from build123d import *

# Parameters (mm, degrees)
SKETCH1_W               = 350
SKETCH1_H               = 175
BOSS_EXTRUDE1_DEPTH     = 6
SKETCH3_W               = 6
SKETCH3_H               = 25
CUT_EXTRUDE1_DEPTH      = 392.357892472
LPATTERN1_COUNT         = 4
LPATTERN1_PITCH         = 50
SKETCH4_W               = 6
SKETCH4_H               = 10
CUT_EXTRUDE2_DEPTH      = 392.357892472
LPATTERN2_COUNT         = 2
LPATTERN2_PITCH         = 165
SKETCH5_W               = 6
SKETCH5_H               = 10
CUT_EXTRUDE3_DEPTH      = 392.357892472
LPATTERN3_COUNT         = 2
LPATTERN3_PITCH         = 165
SKETCH6_W               = 6
SKETCH6_H               = 50
CUT_EXTRUDE4_DEPTH      = 10
SKETCH7_W               = 20
SKETCH7_H               = 10
CUT_EXTRUDE5_DEPTH      = 10
LPATTERN4_COUNT         = 2
LPATTERN4_PITCH         = 165
SKETCH8_R               = 2.5
CUT_EXTRUDE6_DEPTH      = 10
SKETCH9_W               = 10
SKETCH9_H               = 20
CUT_EXTRUDE7_DEPTH      = 10
MIRROR1_COPY_1_SKETCH_W = 6
MIRROR1_COPY_1_SKETCH_H = 25
MIRROR1_COPY_1_DEPTH    = 392.357892472
MIRROR1_COPY_2_SKETCH_W = 6
MIRROR1_COPY_2_SKETCH_H = 25
MIRROR1_COPY_2_DEPTH    = 392.357892472
MIRROR1_COPY_3_SKETCH_W = 6
MIRROR1_COPY_3_SKETCH_H = 25
MIRROR1_COPY_3_DEPTH    = 392.357892472
MIRROR1_COPY_4_SKETCH_W = 6
MIRROR1_COPY_4_SKETCH_H = 10
MIRROR1_COPY_4_DEPTH    = 392.357892472
MIRROR1_COPY_5_SKETCH_W = 6
MIRROR1_COPY_5_SKETCH_H = 10
MIRROR1_COPY_5_DEPTH    = 392.357892472


with BuildPart() as part:
    # Sketch1 → Boss-Extrude1 (new body)
    with BuildSketch(Plane(origin=(0, 0, 0), x_dir=(0, 0, -1), z_dir=(1, 0, 0))):
        with Locations((-175, 87.5)):
            Rectangle(SKETCH1_W, SKETCH1_H)
    extrude(amount=BOSS_EXTRUDE1_DEPTH)

    # Sketch3 → Cut-Extrude1 (cut, through all)
    with BuildSketch(Plane(origin=(6, 0, 0), x_dir=(0, 0, -1), z_dir=(1, 0, 0))):
        with Locations((-297, 162.5)):
            Rectangle(SKETCH3_W, SKETCH3_H)
    cut_extrude1 = extrude(amount=-CUT_EXTRUDE1_DEPTH, mode=Mode.SUBTRACT)

    # LPattern1: Cut-Extrude1 ×4
    with Locations(*[(0, -i * LPATTERN1_PITCH, 0) for i in range(1, LPATTERN1_COUNT)]):
        add(cut_extrude1, mode=Mode.SUBTRACT)

    # Sketch4 → Cut-Extrude2 (cut, through all)
    with BuildSketch(Plane(origin=(6, 0, 0), x_dir=(0, 0, -1), z_dir=(1, 0, 0))):
        with Locations((-279, 170)):
            Rectangle(SKETCH4_W, SKETCH4_H)
    cut_extrude2 = extrude(amount=-CUT_EXTRUDE2_DEPTH, mode=Mode.SUBTRACT)

    # LPattern2: Cut-Extrude2 ×2
    with Locations(*[(0, -i * LPATTERN2_PITCH, 0) for i in range(1, LPATTERN2_COUNT)]):
        add(cut_extrude2, mode=Mode.SUBTRACT)

    # Sketch5 → Cut-Extrude3 (cut, through all)
    with BuildSketch(Plane(origin=(6, 0, 0), x_dir=(0, 0, -1), z_dir=(1, 0, 0))):
        with Locations((-249, 170)):
            Rectangle(SKETCH5_W, SKETCH5_H)
    cut_extrude3 = extrude(amount=-CUT_EXTRUDE3_DEPTH, mode=Mode.SUBTRACT)

    # LPattern3: Cut-Extrude3 ×2
    with Locations(*[(0, -i * LPATTERN3_PITCH, 0) for i in range(1, LPATTERN3_COUNT)]):
        add(cut_extrude3, mode=Mode.SUBTRACT)

    # Sketch6 → Cut-Extrude4 (cut)
    with BuildSketch(Plane(origin=(6, 0, 0), x_dir=(0, 0, -1), z_dir=(1, 0, 0))):
        with Locations((-175, 150)):
            Rectangle(SKETCH6_W, SKETCH6_H)
    extrude(amount=-CUT_EXTRUDE4_DEPTH, mode=Mode.SUBTRACT)

    # Sketch7 → Cut-Extrude5 (cut)
    with BuildSketch(Plane(origin=(6, 0, 0), x_dir=(0, 0, -1), z_dir=(1, 0, 0))):
        with Locations((-212, 170)):
            Rectangle(SKETCH7_W, SKETCH7_H)
    cut_extrude5 = extrude(amount=-CUT_EXTRUDE5_DEPTH, mode=Mode.SUBTRACT)

    # LPattern4: Cut-Extrude5 ×2
    with Locations(*[(0, -i * LPATTERN4_PITCH, 0) for i in range(1, LPATTERN4_COUNT)]):
        add(cut_extrude5, mode=Mode.SUBTRACT)

    # Sketch8 → Cut-Extrude6 (cut)
    with BuildSketch(Plane(origin=(6, 0, 0), x_dir=(0, 0, -1), z_dir=(1, 0, 0))):
        with Locations((-222, 145)):
            Circle(SKETCH8_R)
        with Locations((-202, 145)):
            Circle(SKETCH8_R)
        with Locations((-222, 30)):
            Circle(SKETCH8_R)
        with Locations((-202, 30)):
            Circle(SKETCH8_R)
    extrude(amount=-CUT_EXTRUDE6_DEPTH, mode=Mode.SUBTRACT)

    # Sketch9 → Cut-Extrude7 (cut)
    with BuildSketch(Plane(origin=(6, 0, 0), x_dir=(0, 0, -1), z_dir=(1, 0, 0))):
        with Locations((-305, 10)):
            Rectangle(SKETCH9_W, SKETCH9_H)
    cut_extrude7 = extrude(amount=-CUT_EXTRUDE7_DEPTH, mode=Mode.SUBTRACT)

    # Mirror1: Cut-Extrude1, Cut-Extrude2, Cut-Extrude3, Cut-Extrude7 across plane
    add(cut_extrude1.mirror(Plane.XY.offset(175)), mode=Mode.SUBTRACT)
    add(cut_extrude2.mirror(Plane.XY.offset(175)), mode=Mode.SUBTRACT)
    add(cut_extrude3.mirror(Plane.XY.offset(175)), mode=Mode.SUBTRACT)
    add(cut_extrude7.mirror(Plane.XY.offset(175)), mode=Mode.SUBTRACT)

    # Mirror1 copy 1 sketch → Mirror1 copy 1 (cut, through all)
    with BuildSketch(Plane(origin=(6, -50, 350), x_dir=(0, 0, 1), z_dir=(1, 0, 0))):
        with Locations((-297, -162.5)):
            Rectangle(MIRROR1_COPY_1_SKETCH_W, MIRROR1_COPY_1_SKETCH_H)
    extrude(amount=-MIRROR1_COPY_1_DEPTH, mode=Mode.SUBTRACT)

    # Mirror1 copy 2 sketch → Mirror1 copy 2 (cut, through all)
    with BuildSketch(Plane(origin=(6, -100, 350), x_dir=(0, 0, 1), z_dir=(1, 0, 0))):
        with Locations((-297, -162.5)):
            Rectangle(MIRROR1_COPY_2_SKETCH_W, MIRROR1_COPY_2_SKETCH_H)
    extrude(amount=-MIRROR1_COPY_2_DEPTH, mode=Mode.SUBTRACT)

    # Mirror1 copy 3 sketch → Mirror1 copy 3 (cut, through all)
    with BuildSketch(Plane(origin=(6, -150, 350), x_dir=(0, 0, 1), z_dir=(1, 0, 0))):
        with Locations((-297, -162.5)):
            Rectangle(MIRROR1_COPY_3_SKETCH_W, MIRROR1_COPY_3_SKETCH_H)
    extrude(amount=-MIRROR1_COPY_3_DEPTH, mode=Mode.SUBTRACT)

    # Mirror1 copy 4 sketch → Mirror1 copy 4 (cut, through all)
    with BuildSketch(Plane(origin=(6, -165, 350), x_dir=(0, 0, 1), z_dir=(1, 0, 0))):
        with Locations((-279, -170)):
            Rectangle(MIRROR1_COPY_4_SKETCH_W, MIRROR1_COPY_4_SKETCH_H)
    extrude(amount=-MIRROR1_COPY_4_DEPTH, mode=Mode.SUBTRACT)

    # Mirror1 copy 5 sketch → Mirror1 copy 5 (cut, through all)
    with BuildSketch(Plane(origin=(6, -165, 350), x_dir=(0, 0, 1), z_dir=(1, 0, 0))):
        with Locations((-249, -170)):
            Rectangle(MIRROR1_COPY_5_SKETCH_W, MIRROR1_COPY_5_SKETCH_H)
    extrude(amount=-MIRROR1_COPY_5_DEPTH, mode=Mode.SUBTRACT)


solid = part.part
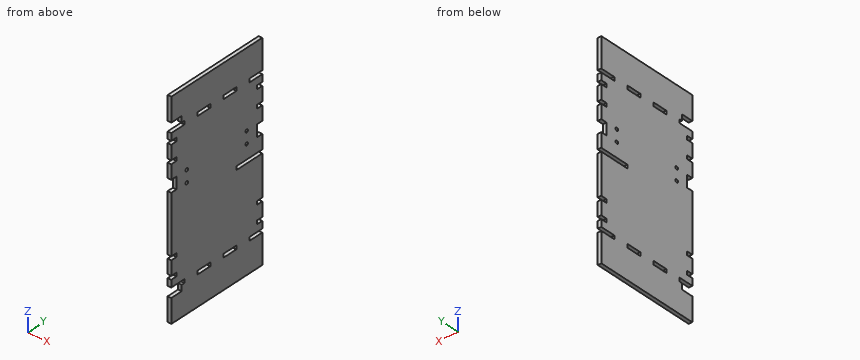
Input: part model. Units: mm. Frame: model coordinates. Coordinates: 2 decimals unless noted, no trailing zeros. Order: outer loops, then holes, each group sorted by start corner. A loop starts at its lowest first (then second) coordinate and runs counter-clockwise, first axis right, second up. Notation, with made-up numbers: M 18,32.25 L 63,32.25 A13 ccw 63,47.25 Z; hole C 67,67.25 d2. An arc over 180 degrees is marked long. Write item = value, one per line. Start each with the question number.
(1) Section B-B on y = 55.5. Output: boundary loops of the cut face in (x, z).
(2) First-contact query: P1, Ø1.8, axis at x = 4.5, z = 212.5, coming from the +Y side; P2, Ø3, axis at x = 4, z = 208, coming from the -Y side; P3, Ø12, axis at y = 113, z = 211, coming from the -X side; P4, Ø1.8, axis at x = 2.5, z = 296, coming from the +Y side. Flat tips, straight axial feed; report the tip coordinate or a pass-through.
(3) Section C-C on x = 1.55. Give the number of separate pieces and of enclosed holes in the cut face, and give its area (3 significant figures).
(4) Section A-A on y = 135. Output: boundary loops of the cut face in (x, z), and give its area (3 significant figures).
(5) Line query: line 1 along Z through (x, y) = (3.35, 18); line 2 along Z through (x, y) = (3.05, 145); line 3 along Z through (x, y) = (4.2, 118). Output: solid intervals per line, ascending. Write a range as [from, to].
Result set:
q1.outline = M 0,0 L 6,0 L 6,50 L 0,50 Z; M 0,56 L 6,56 L 6,294 L 0,294 Z; M 0,300 L 6,300 L 6,350 L 0,350 Z
q2.P1 = 165
q2.P2 = 10
q2.P3 = 0
q2.P4 = 150
q3.separate_pieces = 1
q3.enclosed_holes = 8
q3.area = 58,400 mm²
q4.outline = M 0,0 L 6,0 L 6,172 L 0,172 Z; M 0,178 L 6,178 L 6,350 L 0,350 Z
q4.area = 2,060 mm²
q5.line_1 = [0, 40], [56, 294], [310, 350]
q5.line_2 = [0, 172], [178, 199.5], [204.5, 219.5], [224.5, 350]
q5.line_3 = [0, 50], [56, 294], [300, 350]
